```python
from build123d import *

# Parameters (mm, degrees)
SKETCH_1_R                = 30
EXTRUDE_1_DEPTH           = 20
MM_1_D                    = 6
MM_1_DEPTH                = 20
MM_1_TIP                  = 1.802581857
HOLE_WIZARD_1_D           = 6.6
HOLE_WIZARD_1_DEPTH       = 20
HOLE_WIZARD_1_CBORE_D     = 11
HOLE_WIZARD_1_CBORE_DEPTH = 6.8
HOLE_WIZARD_1_TIP         = 1.982840043
SKETCH_6_OUTSIDE_W        = 79.436
SKETCH_6_OUTSIDE_H        = 79.436
SKETCH_6_OUTSIDE_R        = 21
CUT_EXTRUDE_1_DEPTH       = 15
CHAMFER_1_SIZE            = 8
CHAMFER_1_SIZE2           = 2.911761874
SKETCH_7_W                = 35.972327204
SKETCH_7_H                = 68.406392716
CUT_EXTRUDE_2_DEPTH       = 47.904157598


with BuildPart() as part:
    # 草图1 → 凸台-拉伸1 (new body)
    with BuildSketch(Plane.XY):
        Circle(SKETCH_1_R)
    extrude(amount=EXTRUDE_1_DEPTH)

    # 大小mm 暗销孔1
    with Locations(Plane.XY.offset(20)):
        with Locations((-13, 0), (7, 0)):
            Hole(MM_1_D / 2, depth=MM_1_DEPTH)
            with Locations((0, 0, -(MM_1_DEPTH + MM_1_TIP / 2))):  # 118° drill point
                Cone(0, MM_1_D / 2, MM_1_TIP, mode=Mode.SUBTRACT)

    # 打孔尺寸(%根据)内六角圆柱头螺钉的类型1
    with Locations(Plane.XY.offset(20)):
        with Locations((-3, 0)):
            CounterBoreHole(HOLE_WIZARD_1_D / 2, HOLE_WIZARD_1_CBORE_D / 2, HOLE_WIZARD_1_CBORE_DEPTH, depth=HOLE_WIZARD_1_DEPTH)
            with Locations((0, 0, -(HOLE_WIZARD_1_DEPTH + HOLE_WIZARD_1_TIP / 2))):  # 118° drill point
                Cone(0, HOLE_WIZARD_1_D / 2, HOLE_WIZARD_1_TIP, mode=Mode.SUBTRACT)

    # 草图6 outside → 切除-拉伸1 (cut)
    with BuildSketch(Plane.XY.offset(20)):
        Rectangle(SKETCH_6_OUTSIDE_W, SKETCH_6_OUTSIDE_H)
        Circle(SKETCH_6_OUTSIDE_R, mode=Mode.SUBTRACT)
    extrude(amount=-CUT_EXTRUDE_1_DEPTH, mode=Mode.SUBTRACT)

    # 倒角1
    chamfer_1_edges = [part.edges().sort_by_distance(p)[0] for p in [
        (-21, 0, 20),
    ]]
    chamfer_1_side = [part.faces().sort_by_distance(p)[0] for p in [
        (-21, 0, 12.5),
    ]]
    chamfer(chamfer_1_edges, length=CHAMFER_1_SIZE, length2=CHAMFER_1_SIZE2, reference=chamfer_1_side[0])

    # 草图7 → 切除-拉伸2 (cut, through all)
    with BuildSketch(Plane.XY.offset(20)):
        with Locations((29.986163602, -1.092611915)):
            Rectangle(SKETCH_7_W, SKETCH_7_H)
    extrude(amount=-CUT_EXTRUDE_2_DEPTH, mode=Mode.SUBTRACT)


solid = part.part
```
Verification items for the finished model (mm, model axes). A direction names the side the tool comes from. Give positions to 0.01 mm unless a question says otherwise; leave off trailing zeros. Loops run counter-clockwise (first coordinate to the right, second up) from the corner with the lowest first, then second, coordinate; pieces in that order, holes last.
1. Section check C-C, the plane x = -24. Enter the section's corners in (y, z), then the cut area to 3 significant figures.
2. Set-up check for faces 5 (the flat face through (3, 0, 20)), 6 (the flat face through (1, 0, 13.2)): record each of +Z, -Z, +X, -X, +Y, -Y from which the full face is reachable in a straight line by a thin tool's end or side.
3. Thickness scan on line 1 (Z direction, x = -25, y = 2); line 2 (Y direction, x = 5.5, z = 6); line 3 (Y direction, x = -10.5, z = 15.75). Record the ranges inside material, lowest first.
4. Section check D-D, the plane z = 14.25. Enter the section's corners in (x, y).
5. Section check B-B, the plane z = 2. Enter the section's corners in (x, y), then the cut area to 3 significant figures.
6. Go/stop test with flat-tipped pins: pin 1 Ø6 at (x, z) = (-19.5, 5.5) entering from +Y; pin 2 Ø1.5 at (x, z) = (4, 4.5) entering from +Y; pin 3 Ø10 at (x, z) = (-2, 14) entering from -Y. Record where each tip stops, or that it passes through.
7. Section check A-A, the plane y = 0. Enter the section's corners in (x, z), then the cut area to 3 significant figures.
8. Mould release check, pull along X, two halves, no side actions. Record for faces 1 (the flat face through (12, 0, 8)), 2 (the flat face through (-9, 0, 0)), 3 (the cylindrical face through (-6.15, 0.99, 6.51)), 4 (the cylindrical face through (-29.99, 0.83, 2.46)): released by +X, released by -X, zero draft, split by the parting line, or undercut.
Geometry says:
1. outline: (-18, 0) - (18, 0) - (18, 5) - (-18, 5) - close
1. area: 180 mm2
2. face 5: +Z, +X, -X, +Y, -Y
2. face 6: +Z
3. line 1: z = 0 to 5
3. line 2: y = -20.27 to -2.6, 2.6 to 20.27
3. line 3: y = -16.59 to -1.66, 1.66 to 16.59
4. outline: (12, -16.23) - (12, 16.23) arc R20.18 ccw (long way) to start; hole circle Ø6 at (-13, 0); hole circle Ø11 at (-3, 0); hole circle Ø6 at (7, 0)
5. outline: (12, -27.5) - (12, 27.5) arc R30 ccw (long way) to start; hole circle Ø6 at (-13, 0); hole circle Ø6.6 at (-3, 0); hole circle Ø6 at (7, 0)
5. area: 2,020 mm2
6. pin 1: stops at y = 25.03
6. pin 2: stops at y = 29.82
6. pin 3: stops at y = -21
7. outline: (-30, 0) - (-16, 0) - (-16, 20) - (-18.09, 20) - (-21, 12) - (-21, 5) - (-30, 5) - close; (-10, 0) - (-6.3, 0) - (-6.3, 13.2) - (-8.5, 13.2) - (-8.5, 20) - (-10, 20) - close; (0.3, 0) - (4, 0) - (4, 20) - (2.5, 20) - (2.5, 13.2) - (0.3, 13.2) - close; (10, 0) - (12, 0) - (12, 20) - (10, 20) - close
7. area: 291 mm2
8. face 1: released by +X
8. face 2: zero draft
8. face 3: undercut
8. face 4: split by the parting line
